Build history of the part. All positions in model axes, mm. A direction names the side the tool comes from. Round coordinates to 2 decimals unless told otherwise and drop trailing zeros. Write each loop counter-clockwise with the first axis right and the second up, starting at its lowest first coordinate (ties: lowest second). Pieces come first, ordered by that corner, then holes.
1) Flat gauge pins, fed straight in: pin 1 (10 mm diameter, centred on x = 178.5, z = -35.5, fed in from +Y); pin 2 (8 mm diameter, centred on y = -36, z = -21.5, fed in from -X); pin 3 (2 mm diameter, centred on x = 115.5, z = 1, fed in from +Y). Where does each tip first touch, or does it go through?
2) Saw through at A-A (z = 0). Write the cut outline in (x, y).
3) Saw through at D-D (x = 203). Write the cut outline in (y, z).
4) Pull direction Z, two halves, no side cores. Call faces 4 (the cylindrical face through (250, 30, 0)), 5 (the cylindrical face through (131.835, 42.362, 22.034)), 6 (the flat face through (290, 0, 0)): +Z half, -Z half, draft (parallel to the pull), parting line (faces both ways), or undercut.
5) Wall check: probe 1 along X at (y, z) = (21.5, -36.5); probe 2 along Y at (x, z) = (100.5, -2); probe 3 along Z at (x, y) = (233, 31). Give the ranges that are in metal, low to high.
6) Which spindle directions (+Z, -Z, +X, -X, +Y, -Y) get a long thin tool onto all of the face, cutting with end or side? Do faces 1 (the cylindrical face through (216.975, 34.168, -7.587)), 2 (the flat face through (85, -22, 21)), 3 (the flat face through (222, 30, 5)). Say none if no direction does.
7) Saw through at B-B (y = 0). Write the cut outline in (x, z).
8) Saw through at C-C (x = 64.5). Write the cut outline in (y, z).
from build123d import *

# Parameters (mm, degrees)
CHAFL_N1_SIZE         = 2
CORTAR_EXTRUIR1_DEPTH = 10


with BuildPart() as part:
    # Croquis1 → Revolución1 (revolve)
    with BuildSketch(Plane.XY, mode=Mode.PRIVATE) as revoluci_n1_sk:
        Polygon((0, 0), (290, 0), (290, 30), (255, 30), (255, 35), (180, 35), (180, 47.75), (85, 47.75), (85, 30), (0, 30), align=None)
    revolve(revoluci_n1_sk.sketch.rotate(Axis((0, 0, 0), (1, 0, 0)), 90), axis=Axis((0, 0, 0), (1, 0, 0)))

    # Chaflán1
    chafl_n1_edges = [part.edges().sort_by_distance(p)[0] for p in [
        (290, 0, -30),
        (0, 0, -30),
    ]]
    chamfer(chafl_n1_edges, length=CHAFL_N1_SIZE)

    # Croquis2 → Cortar-Extruir1 (cut)
    with BuildSketch(Plane(origin=(30.68575842, 35, 0), x_dir=(1, 0, 0), z_dir=(0, 1, 0))):
        with BuildLine():
            Line((169.31424158, -5), (214.31424158, -5))
            ThreePointArc((214.31424158, -5), (219.31424158, 0), (214.31424158, 5))
            Line((214.31424158, 5), (169.31424158, 5))
            ThreePointArc((169.31424158, 5), (164.31424158, 0), (169.31424158, -5))
        make_face()
    extrude(amount=-CORTAR_EXTRUIR1_DEPTH, mode=Mode.SUBTRACT)


solid = part.part
Evaluation:
1. pin 1: stops at y = 36.74
1. pin 2: stops at x = 85
1. pin 3: stops at y = 47.75
2. outline: (0, -28) - (2, -30) - (85, -30) - (85, -47.75) - (180, -47.75) - (180, -35) - (255, -35) - (255, -30) - (288, -30) - (290, -28) - (290, 28) - (288, 30) - (255, 30) - (255, 35) - (250, 35) - (250, 25) - (195, 25) - (195, 35) - (180, 35) - (180, 47.75) - (85, 47.75) - (85, 30) - (2, 30) - (0, 28) - close
3. outline: (25, -5) - (25, 5) - (34.64, 5) arc R35 ccw (long way) to (34.64, -5) - close
4. face 4: undercut
4. face 5: parting line
4. face 6: draft
5. probe 1: x = 85 to 180
5. probe 2: y = -47.71 to 47.71
5. probe 3: z = -16.25 to -5, 5 to 16.25
6. face 1: +X
6. face 2: -X
6. face 3: +Y
7. outline: (0, -28) - (2, -30) - (85, -30) - (85, -47.75) - (180, -47.75) - (180, -35) - (255, -35) - (255, -30) - (288, -30) - (290, -28) - (290, 28) - (288, 30) - (255, 30) - (255, 35) - (180, 35) - (180, 47.75) - (85, 47.75) - (85, 30) - (2, 30) - (0, 28) - close
8. outline: circle Ø60 at (0, 0)
